Geometry check sheet. Reference: the model listing, model coordinates, mm. A direction names the side the tool comes from. Round coordinates to 2 decimals unless told otherwise and drop trailing zeros. Write each loop counter-clockwise with the first axis right and the second up, starting at its lowest first coordinate (ties: lowest second). Pieces come first, ordered by that corner, then holes. Notation, with made-up numbers: (27.25, 57) - (41.25, 57) arc R16 ccw to (41.25, 68) - close; hole circle Ø5 at (72.25, 24.5). An arc over 180 degrees is marked (long way). Return JSON: item names as keys, results as strings.
Autodesk Inventor part; units mm, degrees
ref_plane "YZ Plane" through (0, 0, 0) normal (1, 0, 0) x (0, 1, 0)
ref_plane "XZ Plane" through (0, 0, 0) normal (0, 1, 0) x (-1, 0, 0)
ref_plane "XY Plane" through (0, 0, 0) normal (0, 0, 1) x (1, 0, 0)
sketch "Эскиз1" plane through (0, 0, 0) normal (0, 0, 1) x (1, 0, 0)
  circle A0 centre (0, 0) radius 4.25
  circle A1 centre (0, 0) radius 7
  line L0 (-3.5, 0) -> (3.5, 0)
  line L1 (-3.5, 2.4109) -> (-3.5, -2.4109)
  line L2 (3.5, 2.4109) -> (3.5, -2.4109)
  dimension "d0" = 8.5
  dimension "d1" = 14
  dimension "d2" = 7
extrude "Выдавливание1" add sketch "Эскиз1" along normal blind 2 contours A0 L2 | L1 A0 | A1
properties part number "ANT_SPACER"
(1) Section check B-B, the plane x = 0. Enter the section's corners in (y, z), plus the area to 3 significant figures.
Response values:
{"outline": "(-7, 0) - (-4.25, 0) - (-4.25, 2) - (-7, 2) - close; (4.25, 0) - (7, 0) - (7, 2) - (4.25, 2) - close", "area": "11.0 mm^2"}
(2) Section check C-C, the plane z = 1.6. Enter the section's corners in (x, y), plus the area to 3 significant figures.
Response values:
{"outline": "circle Ø14 at (0, 0); hole (-3.5, -2.41) arc R4.25 ccw to (3.5, -2.41) - (3.5, 2.41) arc R4.25 ccw to (-3.5, 2.41) - close", "area": "102 mm^2"}
(3) Access from +Z, -Z, +X, -X, +Y, -Y to the whole of each face (thin tool, end or side, straight path). Record for faces 1 (the face through (0, -5, 0)), 2 (the face through (-0.06, 4.25, 0.99)).
Response values:
{"face 1": "-Z, +X, -X, +Y, -Y", "face 2": "+Z, -Z"}
(4) Release check for a two-part mould opening along X. For faces 3 (the face through (0, -5, 2)), 4 (the face through (0.06, -4.25, 0.99)), 5 (the face through (6.466, 2.681, 0.986)) record: pulls with the +X half, pulls with the -X half, needs draft (parallel to the pull), parting line crosses it, or undercut.
Response values:
{"face 3": "needs draft", "face 4": "undercut", "face 5": "parting line crosses it"}
(5) Material ranges on line 1 along X through (y, z) = (0.25, 1.45); line 2 along Y through (x, z) = (-1, 0.75); line 3 along X through (y, z) = (-1.5, 0.5), recorded low to high. Write a range as [from, to].
Response values:
{"line 1": "x = [-7, -3.5], [3.5, 7]", "line 2": "y = [-6.93, -4.13], [4.13, 6.93]", "line 3": "x = [-6.84, -3.5], [3.5, 6.84]"}
(6) Section check A-A, the plane y = 0. Enter the section's corners in (x, z).
Response values:
{"outline": "(-7, 0) - (-3.5, 0) - (-3.5, 2) - (-7, 2) - close; (3.5, 0) - (7, 0) - (7, 2) - (3.5, 2) - close"}
